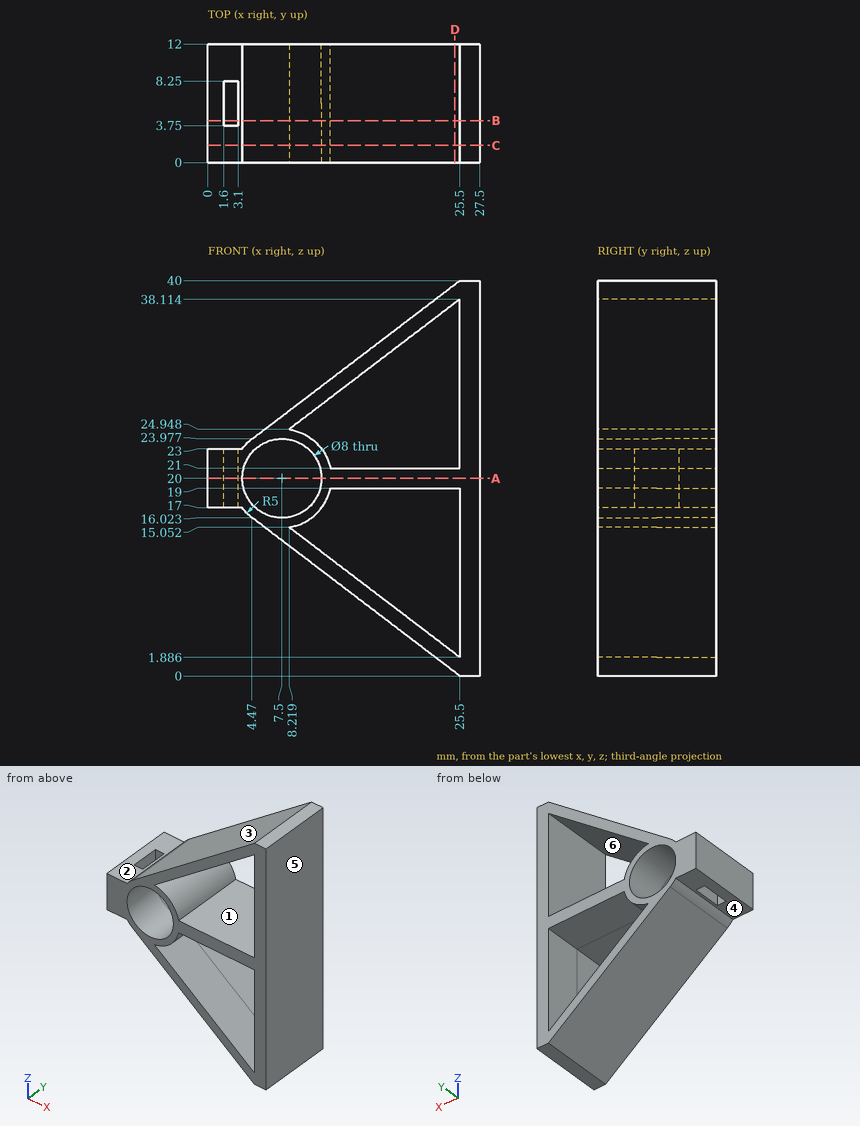
Answer from the drawing. Dimensions are ordinates in mm from the lowest x, y and z of the part. A direction names the side the tool comes from. Round coordinates to 2 decimals unless told otherwise and drop trailing zeros. Loops run counter-clockwise (first coordinate to the right, second up) from the corner with the lowest first, then second, coordinate; pieces in that order, holes last.
(1) The mould has two halves that part along X. Classify the marked faces 1, 2 and 3: pulls with the +X half, pulls with the -X half, needs draft (parallel to the pull), parting line crosses it, or undercut.
Computed values:
face 1: undercut
face 2: needs draft
face 3: pulls with the -X half
(2) Find the intervals of material crossed by L1, parallel to X at y = 7.8, z = 20; L2, parallel to X at y = 10.4, z = 20; L3, parallel to Z at x = 19.25, y = 5.25, in increasing order.
Computed values:
L1: x = 0 to 1.6, 3.1 to 3.5, 11.5 to 27.5
L2: x = 0 to 3.5, 11.5 to 27.5
L3: z = 4.76 to 6.65, 19 to 21, 33.35 to 35.24
(3) Each of these flat-tipped pins is pushed along its axis until it touches: P1, Ø6, axis at x = 14.5, y = 8, coming from the +Z side (1 decimal); P2, Ø4, axis at x = 10.5, y = 10, coming from the +Z side (1 decimal); P3, Ø3, axis at x = 1, y = 3, coming from the -Z side. Where does it stop, or does it pass through?
Computed values:
P1: stops at z = 33.9
P2: stops at z = 30.1
P3: stops at z = 17
(4) For the marked faces 4, 5 and 6, determine the directions among +Z, -Z, +X, -X, +Y, -Y from which every point of the face is accessible in a straight line to the end or side of a thin tool.
Computed values:
face 4: -Z, -X, +Y, -Y
face 5: +Z, -Z, +X, +Y, -Y
face 6: +Y, -Y
(5) The part is cut by section C-C, the plane y = 1.75. Give the vertices of the cut face in (x, z).
Computed values:
outline: (0, 17) - (3.5, 17) arc R5 ccw to (4.47, 16.02) - (25.5, 0) - (27.5, 0) - (27.5, 40) - (25.5, 40) - (4.47, 23.98) arc R5 ccw to (3.5, 23) - (0, 23) - close; hole circle Ø8 at (7.5, 20); hole (8.22, 15.05) - (25.5, 1.89) - (25.5, 19) - (12.4, 19) arc R5 cw to start; hole (8.22, 24.95) arc R5 cw to (12.4, 21) - (25.5, 21) - (25.5, 38.11) - close
(6) The part is cut by section B-B, the plane y = 4.25. Give the vertices of the cut face in (x, z).
Computed values:
outline: (0, 17) - (1.6, 17) - (1.6, 23) - (0, 23) - close; (3.1, 17) - (3.5, 17) arc R5 ccw to (4.47, 16.02) - (25.5, 0) - (27.5, 0) - (27.5, 40) - (25.5, 40) - (4.47, 23.98) arc R5 ccw to (3.5, 23) - (3.1, 23) - close; hole circle Ø8 at (7.5, 20); hole (8.22, 15.05) - (25.5, 1.89) - (25.5, 19) - (12.4, 19) arc R5 cw to start; hole (8.22, 24.95) arc R5 cw to (12.4, 21) - (25.5, 21) - (25.5, 38.11) - close
(7) The part is cut by section A-A, the plane z = 20. Give the vertices of the cut face in (x, y).
Computed values:
outline: (0, 0) - (3.5, 0) - (3.5, 12) - (0, 12) - close; (11.5, 0) - (27.5, 0) - (27.5, 12) - (11.5, 12) - close; hole (1.6, 3.75) - (3.1, 3.75) - (3.1, 8.25) - (1.6, 8.25) - close
(8) The part is cut by section D-D, the plane x = 25. Give the vertices of the cut face in (y, z).
Computed values:
outline: (0, 0.38) - (12, 0.38) - (12, 2.27) - (0, 2.27) - close; (0, 19) - (12, 19) - (12, 21) - (0, 21) - close; (0, 37.73) - (12, 37.73) - (12, 39.62) - (0, 39.62) - close
